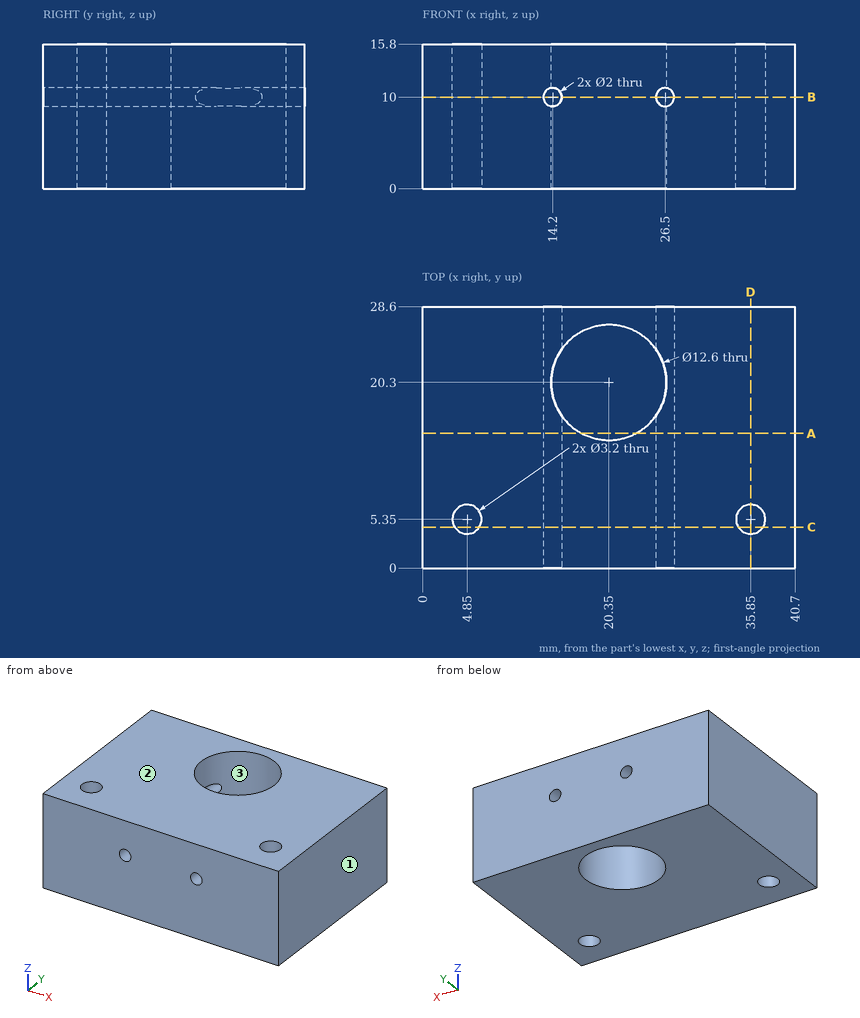
Drawing for the job (mm, zero at the part's lowest x, y, z). Give positions to 0.01 mm unless a question says otherwise; leave off trailing zeros. Order: outer loops, then holes, each group sorted by start corner. A loop starts at its lowest first (then second) coordinate and runs counter-clockwise, first axis right, second up. Notation, with made-up numbers: M 41.5,9 L 55.5,9 A14 ccw 55.5,15 Z; hole C 40,-40 d11. An arc over 180 degrees is marked long. Put each result on its own line as item: value.
Item 1: Slice it at C-C, the plane y = 4.5. Write the cut outline in (x, z).
From the geometry:
outline: M 0,0 L 3.49,0 L 3.49,15.8 L 0,15.8 Z; M 6.21,0 L 34.49,0 L 34.49,15.8 L 6.21,15.8 Z; M 37.21,0 L 40.7,0 L 40.7,15.8 L 37.21,15.8 Z; hole C 14.2,10 d2; hole C 26.5,10 d2
Item 2: Probe line 1 (X direction, y = 10, z = 10); line 2 (Y direction, x = 20.35, z = 12.25); line 3 (X direction, y = 6.5, z = 10). List the from-to ranges inside material, lowest first. Write a range as [from, to].
From the geometry:
line 1: x = [0, 13.2], [15.2, 25.5], [27.5, 40.7]
line 2: y = [0, 14], [26.6, 28.6]
line 3: x = [0, 3.74], [5.96, 13.2], [15.2, 25.5], [27.5, 34.74], [36.96, 40.7]
Item 3: Slice it at A-A, the plane y = 14.75. Write the cut outline in (x, z).
From the geometry:
outline: M 0,0 L 17.37,0 L 17.37,15.8 L 0,15.8 Z; M 23.33,0 L 40.7,0 L 40.7,15.8 L 23.33,15.8 Z; hole C 14.2,10 d2; hole C 26.5,10 d2
Item 4: Two-plate mould, pull along X, no slides. Class the marked faces 1, 2 and 3: +X half, -X half, draft (parallel to the pull), parting line (faces both ways), or undercut.
From the geometry:
face 1: +X half
face 2: draft
face 3: undercut
Item 5: Slice it at B-B, the plane z = 10. Write the cut outline in (x, y), plus the area to 3 significant figures.
From the geometry:
outline: M 0,0 L 13.2,0 L 13.2,28.6 L 0,28.6 Z; M 15.2,0 L 25.5,0 L 25.5,16.67 A6.3 cw 15.2,16.67 Z; M 15.2,23.93 A6.3 cw 25.5,23.93 L 25.5,28.6 L 15.2,28.6 Z; M 27.5,0 L 40.7,0 L 40.7,28.6 L 27.5,28.6 Z; hole C 4.85,5.35 d3.2; hole C 35.85,5.35 d3.2
area: 920 mm2
Item 6: Slice it at D-D, the plane x = 35.85. Write the cut outline in (y, z), plus the area to 3 significant figures.
From the geometry:
outline: M 0,0 L 3.75,0 L 3.75,15.8 L 0,15.8 Z; M 6.95,0 L 28.6,0 L 28.6,15.8 L 6.95,15.8 Z
area: 401 mm2
